CAD build for the part. Positions are in the model's coordinates, mm. A direction names the side the tool comes from. Give positions to 0.01 mm unless a question says otherwise; leave off trailing zeros. Write each loop counter-clockwise with the first axis right and the second up, starting at its lowest first coordinate (ties: lowest second). Pieces come first, ordered by that corner, then holes. Notation, with made-up numbers: (23, -26.75) -> (66, -26.75) arc R29 ccw to (66, 8.25) -> close; hole circle Ø5 at (62.25, 14). An arc over 180 degrees is marked (long way). Answer as a JSON object with one key per item and string values.
```python
from build123d import *

# Parameters (mm, degrees)
PAD_DEPTH       = 30
SKETCH001_R     = 2.75
SKETCH001_R_2   = 6.5
POCKET_DEPTH    = 20.001
POCKET002_DEPTH = 11
POCKET003_DEPTH = 15
POCKET004_DEPTH = 2
POCKET005_DEPTH = 5
POCKET006_DEPTH = 5
POCKET007_DEPTH = 4
CHAMFER_SIZE    = 1
CHAMFER004_SIZE = 2


with BuildPart() as part:
    # Sketch → Pad (new body, symmetric)
    with BuildSketch(Plane.XZ):
        Polygon((0, 0), (0, 20), (60, 20), (80, 0), align=None)
    extrude(amount=PAD_DEPTH, both=True)

    # Sketch001 → Pocket (cut, through all)
    with BuildSketch(Plane.XY):
        with Locations((25, 20)):
            Circle(SKETCH001_R)
        with Locations((25, -20)):
            Circle(SKETCH001_R)
        with Locations((50, 18)):
            Circle(SKETCH001_R_2)
        with Locations((50, -1)):
            Circle(SKETCH001_R_2)
    extrude(amount=POCKET_DEPTH, mode=Mode.SUBTRACT)

    # Sketch003 → Pocket002 (cut)
    with BuildSketch(Plane.XY.offset(20)):
        with BuildLine():
            ThreePointArc((56.5, 26.5), (56.207107, 27.207107), (55.5, 27.5))
            Line((3.5, 27.5), (55.5, 27.5))
            ThreePointArc((3.5, 27.5), (2.792893, 27.207107), (2.5, 26.5))
            Line((2.5, -26.5), (2.5, 26.5))
            ThreePointArc((2.5, -26.5), (2.792893, -27.207107), (3.5, -27.5))
            Line((55.5, -27.5), (3.5, -27.5))
            ThreePointArc((55.5, -27.5), (56.207107, -27.207107), (56.5, -26.5))
            Line((56.5, 26.5), (56.5, -26.5))
        make_face()
    extrude(amount=-POCKET002_DEPTH, mode=Mode.SUBTRACT)

    # Sketch004 → Pocket003 (cut)
    with BuildSketch(Plane.XY.offset(20)):
        with BuildLine():
            ThreePointArc((3.5, 27.5), (2.792893, 27.207107), (2.5, 26.5))
            Line((2.5, -26.5), (2.5, 26.5))
            ThreePointArc((2.5, -26.5), (2.792893, -27.207107), (3.5, -27.5))
            Line((11.5, -27.5), (3.5, -27.5))
            ThreePointArc((11.5, -27.5), (12.207107, -27.207107), (12.5, -26.5))
            Line((12.5, 26.5), (12.5, -26.5))
            ThreePointArc((12.5, 26.5), (12.207107, 27.207107), (11.5, 27.5))
            Line((3.5, 27.5), (11.5, 27.5))
        make_face()
    extrude(amount=-POCKET003_DEPTH, mode=Mode.SUBTRACT)

    # Sketch005 → Pocket004 (cut)
    with BuildSketch(Plane.XY):
        with BuildLine():
            ThreePointArc((2.5, 26.5), (1.792893, 26.207107), (1.5, 25.5))
            Line((1.5, -25.5), (1.5, 25.5))
            ThreePointArc((1.5, -25.5), (1.792893, -26.207107), (2.5, -26.5))
            Line((75.5, -26.5), (2.5, -26.5))
            ThreePointArc((75.5, -26.5), (76.207107, -26.207107), (76.5, -25.5))
            Line((76.5, 25.5), (76.5, -25.5))
            ThreePointArc((76.5, 25.5), (76.207107, 26.207107), (75.5, 26.5))
            Line((2.5, 26.5), (75.5, 26.5))
        make_face()
    extrude(amount=POCKET004_DEPTH, mode=Mode.SUBTRACT)

    # Sketch006 → Pocket005 (cut)
    with BuildSketch(Plane.YZ):
        with BuildLine():
            ThreePointArc((-4.25, 8.261387), (-1, 6.75), (2.25, 8.261387))
            Line((2.25, 21), (2.25, 8.261387))
            Line((-4.25, 21), (2.25, 21))
            Line((-4.25, 8.261387), (-4.25, 21))
        make_face()
        with BuildLine():
            ThreePointArc((14.75, 8.261387), (18, 6.75), (21.25, 8.261387))
            Line((21.25, 21), (21.25, 8.261387))
            Line((14.75, 21), (21.25, 21))
            Line((14.75, 8.261387), (14.75, 21))
        make_face()
        with BuildLine():
            ThreePointArc((-20.25, 11), (-17, 7.75), (-13.75, 11))
            Line((-13.75, 21), (-13.75, 11))
            Line((-20.25, 21), (-13.75, 21))
            Line((-20.25, 11), (-20.25, 21))
        make_face()
    extrude(amount=POCKET005_DEPTH, mode=Mode.SUBTRACT)

    # Sketch007 → Pocket006 (cut)
    with BuildSketch(Plane.XZ.offset(30)):
        with BuildLine():
            ThreePointArc((30, 14), (26, 10), (30, 6))
            Line((30, 6), (45, 6))
            ThreePointArc((45, 6), (49, 10), (45, 14))
            Line((45, 14), (30, 14))
        make_face()
    extrude(amount=-POCKET006_DEPTH, mode=Mode.SUBTRACT)

    # Sketch009 → Pocket007 (cut)
    with BuildSketch(Plane.XZ.offset(25)):
        with BuildLine():
            ThreePointArc((25, 16), (19, 10), (25, 4))
            Line((25, 4), (50, 4))
            ThreePointArc((50, 4), (56, 10), (50, 16))
            Line((50, 16), (25, 16))
        make_face()
    extrude(amount=POCKET007_DEPTH, mode=Mode.SUBTRACT)

    # Chamfer
    chamfer_edges = [part.edges().sort_by_distance(p)[0] for p in [
        (0, -30, 10),
        (0, 30, 10),
        (2.5, -20.25, 15.5),
        (70, 30, 10),
    ]]
    chamfer(chamfer_edges, length=CHAMFER_SIZE)

    # Chamfer004
    chamfer004_edges = [part.edges().sort_by_distance(p)[0] for p in [
        (37.5, -25, 9),
    ]]
    chamfer(chamfer004_edges, length=CHAMFER004_SIZE)


solid = part.part
```
1) Slice it at D-D (z = 10). State how many separate pieces and enclosed holes the cut face has, then the cut area to 3 significant figures.
Model answer:
{"separate pieces": "4", "enclosed holes": "0", "area": "1,100 mm2"}
2) Slice it at B-B (y = 1). List the corners of the cut face in (x, z), then the cut area to 3 significant figures.
Model answer:
{"outline": "(0, 0) -> (1.5, 0) -> (1.5, 2) -> (43.82, 2) -> (43.82, 9) -> (12.5, 9) -> (12.5, 5) -> (2.5, 5) -> (2.5, 7.25) -> (0, 7.25) -> close; (56.18, 2) -> (76.5, 2) -> (76.5, 0) -> (80, 0) -> (60, 20) -> (56.5, 20) -> (56.5, 9) -> (56.18, 9) -> close", "area": "498 mm2"}
3) 3-axis set-ups, long thin cutter, end or side, ignore diameter. For faces 1 (the flat face through (12.5, 0, 7)), 2 (the cylindrical face through (22.253, -19.879, 5.451)), 3 (the flat face through (1, 21.25, 14)): which of +Z, -Z, +X, -X, +Y, -Y reach the whole face in a straight line?
Model answer:
{"face 1": "+Z", "face 2": "+Z, -Z", "face 3": "+Z, -X"}
4) Slice it at C-C (y = 20). List the corners of the cut face in (x, z), then the cut area to 3 significant figures.
Model answer:
{"outline": "(0, 0) -> (1.5, 0) -> (1.5, 2) -> (22.25, 2) -> (22.25, 9) -> (12.5, 9) -> (12.5, 5) -> (2.5, 5) -> (2.5, 7.25) -> (0, 7.25) -> close; (27.75, 2) -> (43.82, 2) -> (43.82, 9) -> (27.75, 9) -> close; (56.18, 2) -> (76.5, 2) -> (76.5, 0) -> (80, 0) -> (60, 20) -> (56.5, 20) -> (56.5, 9) -> (56.18, 9) -> close", "area": "459 mm2"}
5) Wall check: probe 1 along Y at (x, z) = (50, 4.25); probe 2 along Y at (x, z) = (25, 6); probe 3 along X at (y, z) = (20, 6.5). Give the ranges that are in metal, low to high.
Model answer:
{"probe 1": "y = -30 to -29, -25 to -7.5, 5.5 to 11.5, 24.5 to 30", "probe 2": "y = -30 to -29, -25 to -22.75, -17.25 to 17.25, 22.75 to 30", "probe 3": "x = 0 to 2.5, 12.5 to 22.25, 27.75 to 43.82, 56.18 to 73.5"}
6) Pin check, flat tips, straight feed: pin 1 (12 mm diameter, centred on x = 66.5, y = 20, fed in from -Z); pin 2 (1.2 mm diameter, centred on x = 41, y = -26.5, fed in from +Z); pin 3 (22.5 mm diameter, centred on x = 28, y = 10.5, fed in from +Z). Stop position of each tip, or through.
Model answer:
{"pin 1": "stops at z = 2", "pin 2": "stops at z = 4", "pin 3": "stops at z = 9"}
7) Mould opens along X. For faces 4 (the cylindrical face through (1.23, -1.05, 6.75)), 5 (the flat face through (38, 0, 2)), 6 (the flat face through (70, -1, 10)), 7 (the flat face through (24, -27.5, 18)) say: released by +X, released by -X, zero draft, split by the parting line, or undercut.
Model answer:
{"face 4": "zero draft", "face 5": "undercut", "face 6": "released by +X", "face 7": "undercut"}
8) Slice it at A-A (x = 42.5). List the corners of the cut face in (y, z), then the cut area to 4 significant figures.
Model answer:
{"outline": "(-30, 0) -> (-26.5, 0) -> (-26.5, 2) -> (26.5, 2) -> (26.5, 0) -> (30, 0) -> (30, 20) -> (27.5, 20) -> (27.5, 9) -> (-23, 9) -> (-25, 7) -> (-25, 4) -> (-29, 4) -> (-29, 6) -> (-30, 6) -> close; (-30, 14) -> (-29, 14) -> (-29, 16) -> (-27.5, 16) -> (-27.5, 20) -> (-30, 20) -> close", "area": "448.5 mm2"}
